```python
from build123d import *

# Parameters (mm, degrees)
SKETCH1_W           = 20
SKETCH1_H           = 20
SKETCH1_W_2         = 16
SKETCH1_H_2         = 16
BOSS_EXTRUDE1_DEPTH = 100
SKETCH4_R           = 2.5
CUT_EXTRUDE2_DEPTH  = 103.46950766
SKETCH5_W           = 20
SKETCH5_H           = 20
SKETCH5_W_2         = 16
SKETCH5_H_2         = 16
BOSS_EXTRUDE2_DEPTH = 12.3
BOSS_EXTRUDE3_DEPTH = 20
SKETCH7_W           = 16
SKETCH7_H           = 16
CUT_EXTRUDE3_DEPTH  = 114.186969215
CUT_EXTRUDE4_DEPTH  = 103.46950766


with BuildPart() as part:
    # Sketch1 → Boss-Extrude1 (new body)
    with BuildSketch(Plane.XY):
        Rectangle(SKETCH1_W, SKETCH1_H)
        Rectangle(SKETCH1_W_2, SKETCH1_H_2, mode=Mode.SUBTRACT)
    extrude(amount=BOSS_EXTRUDE1_DEPTH)

    # Sketch4 → Cut-Extrude2 (cut, through all)
    with BuildSketch(Plane(origin=(10, 0, 0), x_dir=(0, 0, -1), z_dir=(1, 0, 0))):
        with Locations((-90, 0)):
            Circle(SKETCH4_R)
        with Locations((-75, 0)):
            Circle(SKETCH4_R)
        with Locations((-5, 0)):
            Circle(SKETCH4_R)
        with Locations((-20, 0)):
            Circle(SKETCH4_R)
    extrude(amount=-CUT_EXTRUDE2_DEPTH, mode=Mode.SUBTRACT)

    # Sketch5 → Boss-Extrude2 (add)
    with BuildSketch(Plane(origin=(0, 0, 0), x_dir=(-1, 0, 0), z_dir=(0, 0, -1))):
        Rectangle(SKETCH5_W, SKETCH5_H)
        Rectangle(SKETCH5_W_2, SKETCH5_H_2, mode=Mode.SUBTRACT)
    extrude(amount=BOSS_EXTRUDE2_DEPTH)

    # Sketch6 → Boss-Extrude3 (add)
    with BuildSketch(Plane.ZY.offset(10)):
        Polygon((-12.3, 10), (-12.3, 1.5), (-17.207477288, 10), align=None)
    extrude(amount=-BOSS_EXTRUDE3_DEPTH)

    # Sketch7 → Cut-Extrude3 (cut, through all)
    with BuildSketch(Plane.XY.offset(-12.3)):
        Rectangle(SKETCH7_W, SKETCH7_H)
    extrude(amount=-CUT_EXTRUDE3_DEPTH, mode=Mode.SUBTRACT)

    # Sketch8 → Cut-Extrude4 (cut, through all)
    with BuildSketch(Plane.ZY.offset(10)):
        Polygon((-17.207477288, 10), (-5.660471904, -10), (-17.207477288, -10), align=None)
    extrude(amount=-CUT_EXTRUDE4_DEPTH, mode=Mode.SUBTRACT)


solid = part.part
```
CAD build for the part. Positions are in the model's coordinates, mm. A direction names the side the tool comes from. Give positions to 0.01 mm unless a question says otherwise; leave off trailing zeros. Write each loop counter-clockwise with the first axis right and the second up, starting at its lowest first coordinate (ties: lowest second). Pieces come first, ordered by that corner, then holes. Notation, with made-up numbers: M -24,-19.5 L -8,-19.5 A28 ccw -8,6.5 Z; hole C 36.25,20.25 d3. An arc over 180 degrees is marked long. Return JSON: item names as keys, results as strings. Group by question number.
(1) Mould opens along Z. For faces 1 (the face through (0, -8, 47)), 2 (the face through (-8.986, 0.751, 2.615)), 3 (the face through (-9, 0, 100)) say: pulls with the +Z half, pulls with the -Z half, needs draft (parallel to the pull), parting line crosses it, or undercut.
(2) Drill centre lines: L1, parallel to Y at x = -9.3, z = 90; L2, parallel to X at y = -4.5, z = 55. Where is each one in solid material? Low to high. Write a range as [from, to].
(3) Band-saw the part on B-B (x = 3). Give the cut face in (y, z), and give its area (3 significant figures).
(4) 3-axis set-ups, long thin cutter, end or side, ignore diameter. For faces 4 (the face through (-8, 0, 43)), 5 (the face through (9, 0.1, 22.5)): which of +Z, -Z, +X, -X, +Y, -Y reach the whole face in a straight line?
(5) Band-saw the part on C-C (y = -6.5). Give the cut face in (x, z), and give its area (3 significant figures).
(6) Band-saw the part on D-D (y = 0). State how many separate pieces and enclosed holes the cut face has, and give its area (3 significant figures).
(7) Flat gauge pin, fed straight in: pin 1 Ø3 at (y, z) = (0, 90) entering from -X. Where does the tip first touch, or does it go through?
(8) Band-saw the part on A-A (z = 75). Give the cut face in (x, y).
Entries:
{
 "1": {"face 1": "needs draft", "face 2": "undercut", "face 3": "pulls with the +Z half"},
 "2": {"L1": "y = [-10, -2.5], [2.5, 10]", "L2": "x = [-10, -8], [8, 10]"},
 "3": {"outline": "M -10,-5.66 L -8,-6.82 L -8,100 L -10,100 Z; M 8,-16.05 L 10,-17.21 L 10,100 L 8,100 Z", "area": "446 mm^2"},
 "4": {"face 4": "+Z, -Z", "face 5": "+X, -X"},
 "5": {"outline": "M -10,-7.68 L -8,-7.68 L -8,100 L -10,100 Z; M 8,-7.68 L 10,-7.68 L 10,100 L 8,100 Z", "area": "431 mm^2"},
 "6": {"separate pieces": "10", "enclosed holes": "0", "area": "366 mm^2"},
 "7": {"pin 1": "passes through"},
 "8": {"outline": "M -10,-10 L 10,-10 L 10,-2.5 L 8,-2.5 L 8,-8 L -8,-8 L -8,-2.5 L -10,-2.5 Z; M -10,2.5 L -8,2.5 L -8,8 L 8,8 L 8,2.5 L 10,2.5 L 10,10 L -10,10 Z"}
}
